For this review, take the finished solid that the model builds, in its own axes (mm). Round coordinates to 2 decimals unless told otherwise and drop trailing zeros. Order: outer loops, then holes, each group sorted by start corner. A loop starts at its lowest first (then second) coordinate and runs counter-clockwise, first axis right, second up. Notation, with made-up numbers: (-12, 82) - (29, 82) arc R18 ccw to (29, 90) - close; hole circle Ø7 at (-2, 46.5). An arc over 180 degrees is marked (long way). One line per question, with ' | ' between items.
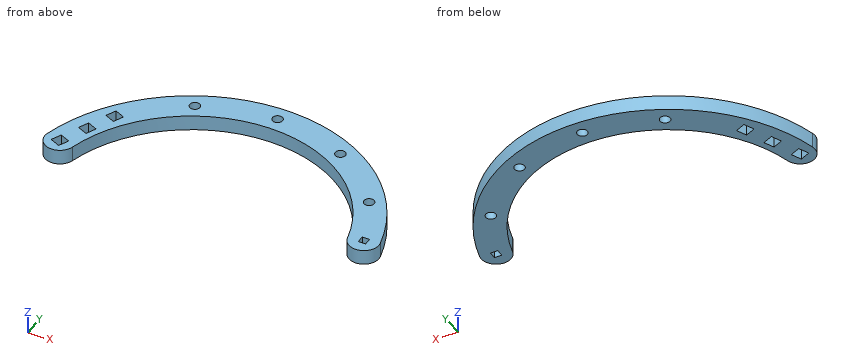
```python
from build123d import *

# Parameters (mm, degrees)
SKETCH2_W           = 3.175
SKETCH2_H           = 3.175
BOSS_EXTRUDE1_DEPTH = 6.35
SKETCH5_R           = 2.1717
CUT_EXTRUDE1_DEPTH  = 25.4


with BuildPart() as part:
    # Sketch2 → Boss-Extrude1 (new body)
    with BuildSketch(Plane.XY):
        with BuildLine():
            ThreePointArc((135.933103671, 1.523612314), (64.8843, 57.15), (-6.164503671, 1.523612314))
            ThreePointArc((-6.164503671, 1.523612314), (-1.523612314, -6.164503671), (6.164503671, -1.523612314))
            ThreePointArc((6.164503671, -1.523612314), (64.8843, 44.45), (123.604096329, -1.523612314))
            ThreePointArc((123.604096329, -1.523612314), (131.292212314, -6.164503671), (135.933103671, 1.523612314))
        make_face()
        Polygon((-1.142495341, 3.111345083), (3.111345083, 1.142495341), (1.142495341, -3.111345083), (-3.111345083, -1.142495341), align=None, mode=Mode.SUBTRACT)
        with Locations((129.7686, 0)):
            Rectangle(SKETCH2_W, SKETCH2_H, mode=Mode.SUBTRACT)
        Polygon((4.191911882, 14.636713109), (2.223061999, 10.38287238), (6.476902727, 8.414022496), (8.445752611, 12.667863225), align=None, mode=Mode.SUBTRACT)
        Polygon((9.526319716, 26.162080852), (7.55746908, 21.9082401), (11.811310114, 19.939390075), (13.780159857, 24.193230498), align=None, mode=Mode.SUBTRACT)
    extrude(amount=BOSS_EXTRUDE1_DEPTH)

    # Sketch5 → Cut-Extrude1 (cut)
    with BuildSketch(Plane(origin=(0, 0, 0), x_dir=(-1, 0, 0), z_dir=(0, 0, -1))):
        with Locations((-64.8843, 50.8)):
            Circle(SKETCH5_R)
        with Locations((-33.823719996, 43.144254616)):
            Circle(SKETCH5_R)
        with Locations((-119.889855449, 21.93085747)):
            Circle(SKETCH5_R)
        with Locations((-95.944880004, 43.144254616)):
            Circle(SKETCH5_R)
    extrude(amount=-CUT_EXTRUDE1_DEPTH, mode=Mode.SUBTRACT)


solid = part.part
```
(1) We need section B-B on z = 3.25. Give the number of separate pieces and of enclosed holes in the cut face, plus the area to 3 significant figures.
Output values:
separate pieces: 1 | enclosed holes: 8 | area: 2,250 mm^2
(2) We need section A-A on y = 39.5. State the section outline as (x, z) points, plus the area to 3 significant figures.
Output values:
outline: (17.22, 0) - (40.92, 0) - (40.92, 6.35) - (17.22, 6.35) - close; (88.85, 0) - (112.55, 0) - (112.55, 6.35) - (88.85, 6.35) - close | area: 301 mm^2
(3) For probe 1 along X at (y, z) = (25.5, 4); probe 2 along X at (y, z) = (14, 1.25); probe 3 along X at (y, z) = (31, 2.75), list the stretches that pass through material, from the lowest coordinate up. Write a range as [from, to].
Output values:
probe 1: [4.63, 9.22], [10.96, 20.91], [108.85, 125.14] | probe 2: [-1.85, 3.9], [5.57, 12.38], [117.39, 131.62] | probe 3: [8.81, 26.86], [102.91, 120.95]
(4) We need section D-D on x = 79.5. State the section outline as (y, z) points, plus the area to 3 significant figures.
Output values:
outline: (42.66, 0) - (55.68, 0) - (55.68, 6.35) - (42.66, 6.35) - close | area: 82.7 mm^2
(5) We need section C-C on y = 50.8. State the section outline as (x, z) points.
Output values:
outline: (35.07, 0) - (62.71, 0) - (62.71, 6.35) - (35.07, 6.35) - close; (67.06, 0) - (94.7, 0) - (94.7, 6.35) - (67.06, 6.35) - close
(6) Insertion check: pin 1 (1 mm diameter, centred on x = 130, z = 4.5, fed in from +Y); pin 2 (3.5 mm diameter, centred on x = 33.82, y = 43.14, fed in from -Z); pin 3 (3 mm diameter, centred on x = 11.5, z = 4, fed in from +Y); pin 4 (3 mm diameter, centred on y = 17, z = 4, fed in from -X). Each pin has a flat end and moves straight along its axis. Give the tip position at first contact, or say it passes through.
Output values:
pin 1: y = 18.33 | pin 2: through | pin 3: y = 35.58 | pin 4: x = -1.16
